Source: CAD feature listing. Evaluate the final solid. Frame: model axes, mm. A direction names the side the tool comes from. Round coordinates to 2 decimals unless told otherwise and drop trailing zeros. Write each loop counter-clockwise with the first axis right and the second up, starting at its lowest first coordinate (ties: lowest second). Pieces come first, ordered by that corner, then holes. Notation, with made-up numbers: M 17.5,-18 L 49.5,-18 A34 cw 49.5,18 Z; hole C 15,6.25 d7. An arc over 180 degrees is marked long. Put each result on its own line as item: value. Start each with the question number.
```python
from build123d import *

# Parameters (mm, degrees)
EXTRUDE_THIN1_DEPTH = 25.4
SKETCH3_R           = 2.14884
CUT_EXTRUDE1_DEPTH  = 26.4
SKETCH4_R           = 2.4892
CUT_EXTRUDE2_DEPTH  = 4.175


with BuildPart() as part:
    # Sketch1 → Extrude-Thin1 (new body)
    with BuildSketch(Plane(origin=(0, 0, 0), x_dir=(1, 0, 0), z_dir=(0, 1, 0))):
        Polygon((0, -25.4), (0, 0), (25.4, 0), (25.4, -3.175), (3.175, -3.175), (3.175, -25.4), align=None)
    extrude(amount=EXTRUDE_THIN1_DEPTH)

    # Sketch3 → Cut-Extrude1 (cut, through all)
    with BuildSketch(Plane(origin=(0, 0, 0), x_dir=(-1, 0, 0), z_dir=(0, 0, -1))):
        with Locations((-8.32866, 12.7)):
            Circle(SKETCH3_R)
        with Locations((-15.33906, 7.10946)):
            Circle(SKETCH3_R)
        with Locations((-15.33906, 18.29054)):
            Circle(SKETCH3_R)
    extrude(amount=-CUT_EXTRUDE1_DEPTH, mode=Mode.SUBTRACT)

    # Sketch4 → Cut-Extrude2 (cut, through all)
    with BuildSketch(Plane(origin=(3.175, 0, 0), x_dir=(0, 0, -1), z_dir=(1, 0, 0))):
        with Locations((-14.2875, 6.35)):
            Circle(SKETCH4_R)
        with Locations((-14.2875, 19.05)):
            Circle(SKETCH4_R)
    extrude(amount=-CUT_EXTRUDE2_DEPTH, mode=Mode.SUBTRACT)


solid = part.part
```
(1) Pull-direction query (Y, two-part tool) for faces 3 (the flat face through (0, 13, 13)), 4 (the flat face through (8, 0, 2)), 5 (the cylindrical face through (17.04, 16.98, 1.57)); classes: +Y half, -Y half, draft (parallel to the pull), parting line (faces both ways), or undercut.
(2) Contact query for flat-ended pins moving along their axis: P1, Ø3, axis at y = 20.5, z = 10, coming from the +X side (3 decimals); P2, Ø6.5, axis at x = 14, y = 12, coming from the +Z side (3 decimals). Output: stop coordinate, or through.
(3) Section query D-D (z = 1.5). Return loops of the section in (x, y).
(4) Section query A-A (y = 12.7). Return loops of the section in (x, z) (1 decimal).
(5) Ray query, line 1 along X through (y, z) = (18.75, 7.75) (3 decimals); line 2 along X through (y, z) = (19.25, 2). Return the intervals inside material, ascending.
(6) Section query B-B (z = 16). Return loops of the section in (x, y) (1 decimal).
(7) Section query C-C (y = 19.5). Return loops of the section in (x, z) (3 decimals), and give its area (3 significant figures).
(8) Access query for faces 1 (the cylindrical face through (1.61, 4.835, 16.263)), 2 (the flat face through (3.175, 13, 14)). Directions: +Z, -Z, +X, -X, +Y, -Y. A direction counts if a zero-diameter tool reaches every point of the face in a straight line with its end or side. Return the directions, or none.
Entries:
1. face 3: draft
1. face 4: -Y half
1. face 5: undercut
2. P1: x = 3.175
2. P2: z = 3.175
3. outline: M 0,0 L 25.4,0 L 25.4,25.4 L 0,25.4 Z; hole C 8.33,12.7 d4.3; hole C 15.34,7.11 d4.3; hole C 15.34,18.29 d4.3
4. outline: M 0,0 L 6.2,0 L 6.2,3.2 L 3.2,3.2 L 3.2,25.4 L 0,25.4 Z; M 10.5,0 L 25.4,0 L 25.4,3.2 L 10.5,3.2 Z
5. line 1: 0 to 3.175
5. line 2: 0 to 13.42, 17.26 to 25.4
6. outline: M 0,0 L 3.2,0 L 3.2,4.5 L 0,4.5 Z; M 0,8.2 L 3.2,8.2 L 3.2,17.2 L 0,17.2 Z; M 0,20.9 L 3.2,20.9 L 3.2,25.4 L 0,25.4 Z
7. outline: M 0,0 L 13.563,0 L 13.563,3.175 L 3.175,3.175 L 3.175,11.839 L 0,11.839 Z; M 0,16.736 L 3.175,16.736 L 3.175,25.4 L 0,25.4 Z; M 17.115,0 L 25.4,0 L 25.4,3.175 L 17.115,3.175 Z
7. area: 124 mm2
8. face 1: +X, -X
8. face 2: +Z, +X, +Y, -Y
